```python
from build123d import *

# Parameters (mm, degrees)
SKETCH2_R           = 2.649999999999999
CUT_EXTRUDE1_DEPTH  = 5
SKETCH5_R           = 2
CUT_EXTRUDE2_DEPTH  = 5
BOSS_EXTRUDE1_START = 10
SKETCH6_R           = 10
SKETCH6_R_2         = 2
BOSS_EXTRUDE1_DEPTH = 10
CUT_EXTRUDE3_DEPTH  = 10
CUT_EXTRUDE4_DEPTH  = 90.00000000000003
FILLET1_R           = 3
CHAMFER1_SIZE       = 1


with BuildPart() as part:
    # Sketch1 → Revolve1 (revolve)
    with BuildSketch(Plane(origin=(0, 0, 0), x_dir=(1, 0, 0), z_dir=(0, 1, 0)), mode=Mode.PRIVATE) as revolve1_sk:
        Polygon((3.65, 0), (3.65, 57.5), (-3.65, 57.5), (-3.65, 49.5), (-0.6499999999999997, 46.5), (-0.6499999999999951, 16.5), (-0.6499999999999819, 12.999999999999988), (-3.650000000000002, 9.999999999999792), (-3.65, 0), align=None)
    revolve(revolve1_sk.sketch.rotate(Axis((-3.65, 0, 0), (1, 0, 0)), 180), axis=Axis((-3.65, 0, 0), (1, 0, 0)))

    # Sketch2 → Cut-Revolve1 (revolve, cut)
    with BuildSketch(Plane(origin=(0, 0, 0), x_dir=(1, 0, 0), z_dir=(0, 1, 0)), mode=Mode.PRIVATE) as cut_revolve1_sk:
        with Locations((0, 57.5)):
            Circle(SKETCH2_R)
    revolve(cut_revolve1_sk.sketch.rotate(Axis((-3.65, 0, 0), (1, 0, 0)), 180), axis=Axis((-3.65, 0, 0), (1, 0, 0)), mode=Mode.SUBTRACT)

    # Sketch4 → Cut-Extrude1 (cut)
    with BuildSketch(Plane(origin=(3.65, 0, 0), x_dir=(0, 0, -1), z_dir=(1, 0, 0))):
        Polygon((7.0725407975729215, 1.73e-15), (3.536270398786459, 6.125000000000007), (-3.536270398786464, 6.125000000000006), (-7.072540797572923, -8.7e-16), (-3.53627039878646, -6.125000000000006), (3.5362703987864603, -6.125000000000006), align=None)
    extrude(amount=-CUT_EXTRUDE1_DEPTH, mode=Mode.SUBTRACT)

    # Sketch5 → Cut-Extrude2 (cut)
    with BuildSketch(Plane.ZY.offset(3.6500000000000012)):
        Circle(SKETCH5_R)
    extrude(amount=-CUT_EXTRUDE2_DEPTH, mode=Mode.SUBTRACT)

    # Sketch6 → Boss-Extrude1 (add)
    with BuildSketch(Plane.ZY.offset(3.6500000000000012).offset(BOSS_EXTRUDE1_START)):
        Circle(SKETCH6_R)
        Circle(SKETCH6_R_2, mode=Mode.SUBTRACT)
    extrude(amount=-BOSS_EXTRUDE1_DEPTH)

    # Sketch7 → Cut-Extrude3 (cut)
    with BuildSketch(Plane(origin=(-1.35, 0, 0), x_dir=(0, 0, -1), z_dir=(1, 0, 0))):
        Polygon((3.5362703987864603, -6.125000000000006), (7.0725407975729215, 1.73e-15), (3.536270398786459, 6.125000000000007), (-3.536270398786464, 6.125000000000006), (-7.072540797572923, -8.7e-16), (-3.53627039878646, -6.125000000000006), align=None)
    extrude(amount=-CUT_EXTRUDE3_DEPTH, mode=Mode.SUBTRACT)

    # Sketch8 → Cut-Extrude4 (cut)
    with BuildSketch(Plane.ZY.offset(0.6499999999999885)):
        with BuildLine():
            Line((14.088457268121097, 11.598076211355), (38.68628497385596, 25.79963865874104))
            ThreePointArc((38.68628497385596, 25.79963865874104), (23.24999999999963, 40.2701812759766), (2.999999999999999, 46.40312489477406))
            Line((2.999999999999999, 46.40312489477406), (3.0000000000000164, 18.00000000000186))
            Line((3.0000000000000164, 18.00000000000186), (3, 17.748239349298846))
            ThreePointArc((3, 17.748239349298846), (8.999999999999696, 15.588457268120239), (13.870426148938957, 11.4721958860035))
            Line((13.870426148938957, 11.4721958860035), (14.088457268121097, 11.598076211355))
        make_face()
        with BuildLine():
            Line((-2.9999999999999827, 18.000000000001936), (-2.999999999999999, 46.40312489477406))
            ThreePointArc((-2.999999999999999, 46.40312489477406), (-23.25000000000001, 40.27018127597639), (-38.68628497385646, 25.799638658740314))
            Line((-38.68628497385646, 25.799638658740314), (-14.08845726812106, 11.598076211354021))
            Line((-14.08845726812106, 11.598076211354021), (-13.870426148939515, 11.472195886002819))
            ThreePointArc((-13.870426148939515, 11.472195886002819), (-9.000000000000009, 15.588457268119885), (-3, 17.748239349298846))
            Line((-3, 17.748239349298846), (-2.9999999999999827, 18.000000000001936))
        make_face()
        with BuildLine():
            Line((17.088457268121093, 6.401923788647327), (41.68628497385644, 20.603486236033717))
            ThreePointArc((41.68628497385644, 20.603486236033717), (46.5, 4.2591e-13), (41.686284973856814, -20.603486236032953))
            Line((41.686284973856814, -20.603486236032953), (17.088457268121957, -6.401923788646879))
            Line((17.088457268121957, -6.401923788646879), (16.870426148939835, -6.276043463295346))
            ThreePointArc((16.870426148939835, -6.276043463295346), (18.000000000000146, 4.3265e-13), (16.870426148939533, 6.276043463296158))
            Line((16.870426148939533, 6.276043463296158), (17.088457268121093, 6.401923788647327))
        make_face()
        with BuildLine():
            Line((14.088457268121054, -11.598076211354028), (38.686284973856445, -25.799638658740335))
            ThreePointArc((38.686284973856445, -25.799638658740335), (23.25000000000037, -40.27018127597618), (3.00000000000084, -46.403124894773995))
            Line((3.00000000000084, -46.403124894773995), (3.0000000000008593, -18.000000000001883))
            Line((3.0000000000008593, -18.000000000001883), (3.000000000000877, -17.748239349298846))
            ThreePointArc((3.000000000000877, -17.748239349298846), (9.000000000000448, -15.588457268119802), (13.87042614893951, -11.472195886002828))
            Line((13.87042614893951, -11.472195886002828), (14.088457268121054, -11.598076211354028))
        make_face()
        with BuildLine():
            Line((-3.0000000000000413, -18.000000000001357), (-2.9999999999999933, -46.40312489477406))
            ThreePointArc((-2.9999999999999933, -46.40312489477406), (-23.24999999999963, -40.2701812759766), (-38.68628497385596, -25.799638658741056))
            Line((-38.68628497385596, -25.799638658741056), (-14.088457268121093, -11.598076211355007))
            Line((-14.088457268121093, -11.598076211355007), (-13.870426148938956, -11.472195886003506))
            ThreePointArc((-13.870426148938956, -11.472195886003506), (-8.999999999999696, -15.588457268120242), (-3.000000000000022, -17.748239349298988))
            Line((-3.000000000000022, -17.748239349298988), (-3.0000000000000413, -18.000000000001357))
        make_face()
        with BuildLine():
            Line((-17.088457268121093, -6.401923788647334), (-41.68628497385644, -20.603486236033735))
            ThreePointArc((-41.68628497385644, -20.603486236033735), (-46.5, -4.2796e-13), (-41.68628497385683, 20.60348623603293))
            Line((-41.68628497385683, 20.60348623603293), (-17.08845726812196, 6.40192378864687))
            Line((-17.08845726812196, 6.40192378864687), (-16.87042614893984, 6.276043463295337))
            ThreePointArc((-16.87042614893984, 6.276043463295337), (-18.000000000000146, -4.4544e-13), (-16.870426148939533, -6.276043463296166))
            Line((-16.870426148939533, -6.276043463296166), (-17.088457268121093, -6.401923788647334))
        make_face()
    extrude(amount=-CUT_EXTRUDE4_DEPTH, mode=Mode.SUBTRACT)

    # Fillet1
    fillet1_edges = [part.edges().sort_by_distance(p)[0] for p in [
        (1.5000000000000058, -11.47219588600283, 13.87042614893951),
        (1.5000000000000058, -25.799638658740335, 38.686284973856445),
        (1.5000000000000058, -46.403124894773995, 3.0000000000008398),
        (1.5000000000000058, -17.74823934929885, 3.0000000000008775),
        (1.5000000000000058, 6.276043463296158, 16.870426148939536),
        (1.5000000000000058, 20.603486236033717, 41.686284973856445),
        (1.5000000000000058, -20.603486236032957, 41.686284973856814),
        (1.5000000000000058, -6.276043463295347, 16.870426148939835),
        (1.5000000000000058, 17.748239349298842, -2.9999999999999982),
        (1.5000000000000058, 11.472195886002819, -13.870426148939515),
        (1.5000000000000058, 25.799638658740314, -38.68628497385646),
        (1.5000000000000058, 46.403124894774066, -2.999999999999999),
        (1.5000000000000058, -6.276043463296168, -16.87042614893953),
        (1.5000000000000058, -20.60348623603374, -41.686284973856445),
        (1.5000000000000058, 20.603486236032932, -41.68628497385683),
        (1.5000000000000058, 6.276043463295337, -16.870426148939835),
        (1.5000000000000058, 17.74823934929885, 3),
        (1.5000000000000058, 46.403124894774066, 3.0000000000000004),
        (1.5000000000000058, 25.799638658741042, 38.68628497385596),
        (1.5000000000000058, 11.472195886003501, 13.870426148938959),
        (1.5000000000000058, -17.748239349298988, -3.0000000000000218),
        (1.5000000000000058, -46.40312489477405, -2.999999999999994),
        (1.5000000000000058, -25.799638658741056, -38.686284973855955),
        (1.5000000000000058, -11.472195886003506, -13.870426148938956),
    ]]
    fillet(fillet1_edges, radius=FILLET1_R)

    # Chamfer1
    chamfer1_edges = [part.edges().sort_by_distance(p)[0] for p in [
        (3.65, -3.062500000000002, -5.304405598179691),
        (3.65, 3.0625000000000044, -5.30440559817969),
        (3.65, 6.125000000000007, 2.66e-15),
        (3.65, 3.0625000000000027, 5.304405598179693),
        (3.65, -3.0625000000000036, 5.304405598179692),
        (3.65, -6.125000000000006, 0),
    ]]
    chamfer(chamfer1_edges, length=CHAMFER1_SIZE)


solid = part.part
```
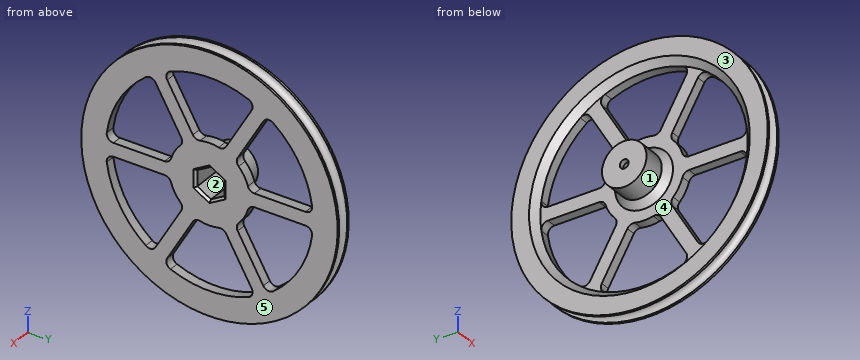
Verification items for the finished model (mm, model axes). Face numbers are marked on the shaded views. A direction names the side the tool comes from. Round coordinates to 2 decimals unless told otherwise and drop trailing zeros. Order: outer loops, then holes, each group sorted by start corner. A loop starts at its lowest first (then second) coordinate and runs counter-clockwise, first axis right, second up. Notation, with made-up numbers: (48.25, 21.25) - (107.25, 21.25) arc R31 ccw to (107.25, 52.25) - close; hole circle Ø7 at (4, 66). An arc over 180 degrees is marked (long way). Use CSV: the item, a comma, the result in double quotes. Start each with the question number.
1) Section check C-C, the plane z = 30. State how many separate pieces and enclosed holes the cut face has, plus the area to 3 significant figures.
2) Section check A-A, the plane z = 0. Record the cut outline in (x, y) (3 decimals), plus the area to 3 significant figures.
3) Section check B-B, the plane x = -6.25. Record the cut outline in (y, z) (3 decimals), plus the area to 3 significant figures.
4) Go/stop test with flat-tipped pins: P1, Ø3.5, axis at x = 2.5, y = 36, coming from the -Z side; P2, Ø8, axis at x = -3.5, z = 12.5, coming from the +Y side; P3, Ø3.5, axis at x = -4, z = -1, coming from the +Y side. Record where each tip stops, or that it passes through.
5) Mould release check, pull along Y, two halves, no side actions. Record for the marked faces 1, 2 and 3: +Y half, -Y half, draft (parallel to the pull), parting line (faces both ways), or undercut.
6) Thickness scan on L1, parallel to Y at x = -12.3, z = 0; L2, parallel to Z at x = 1.5, y = -19; L3, parallel to Z at x = 0.25, y = -38. Record the ranges inside material, lowest first.
7) Access from +Z, -Z, +X, -X, +Y, -Y to the whole of each face (thin tool, end or side, straight path). Record for the marked faces 4 and 5.
Answers:
1,separate pieces,"4"
1,enclosed holes,"0"
1,area,"219 mm²"
2,outline,"(-13.65, -10) - (-3.65, -10) - (-0.65, -13) - (-0.65, -46.5) - (-3.65, -49.5) - (-3.65, -57.5) - (-2.65, -57.5) arc R2.65 cw to (2.65, -57.5) - (3.65, -57.5) - (3.65, -7.125) - (2.65, -6.125) - (-11.35, -6.125) - (-11.35, -2) - (-13.65, -2) - close; (-13.65, 2) - (-11.35, 2) - (-11.35, 6.125) - (2.65, 6.125) - (3.65, 7.125) - (3.65, 57.5) - (2.65, 57.5) arc R2.65 cw to (-2.65, 57.5) - (-3.65, 57.5) - (-3.65, 49.5) - (-0.65, 46.5) - (-0.65, 13) - (-3.65, 10) - (-13.65, 10) - close"
2,area,"604 mm²"
3,outline,"circle Ø20 at (0, 0); hole (-6.125, -3.536) - (0, -7.073) - (6.125, -3.536) - (6.125, 3.536) - (0, 7.073) - (-6.125, 3.536) - close"
3,area,"184 mm²"
4,P1,"stops at z = -46.18"
4,P2,"stops at y = 56.87"
4,P3,"stops at y = 57.5"
5,face 1,"parting line"
5,face 2,"undercut"
5,face 3,"draft"
6,L1,"y = -10 to -2, 2 to 10"
6,L2,"z = -51.95 to -41.71, -38.91 to -26.91, -3.22 to 3.22, 26.91 to 38.91, 41.71 to 51.95"
6,L3,"z = -39.57 to -26.8, -3 to 3, 26.8 to 39.57"
7,face 4,"-X"
7,face 5,"+Z, -Z, +X, +Y, -Y"
